For this review, take the finished solid that the model builds, in its own axes (mm). A direction names the side the tool comes from. Give positions to 0.01 mm unless a question says otherwise; leave off trailing zeros. Write each loop counter-clockwise with the first axis right and the second up, starting at its lowest first coordinate (ties: lowest second). Pieces come first, ordered by that corner, then holes.
Q1. Machinability: for faces 5 (the flat face through (10, -12, 1)), 6 (the flat face through (5, -24, 1)), which of the approach directions +Z, -Z, +X, -X, +Y, -Y give a long, thin tool a straight path to every point of the face, cutting with its end or side? Answer none if there is none.
Q2. We need section B-B (z = 0.95). Write out the cut boundary in (x, y), then the cut area to 3 significant figures.
Q3. Mouldability with a two-part tool opening along Y and no side actions: class faces 1 (the flat face through (36, 14, 1)), 2 (the flat face through (48, 19, 1)), 3 (the cylindrical face through (5.914, -17.567, 1.479)), 4 (the flat face through (24, 24, 1)) as released by +Y, released by -Y, zero draft, split by the parting line, or undercut.
Q4. Insertion check: P1, Ø2.5, axis at x = 5, y = 19, coming from the +Z side; P2, Ø1.5, axis at y = -6.5, z = 1.5, coming from the +X side. Each pin has a flat end and moves straight along its axis. Give the tip position at first contact, or say it passes through.
Q5. We need section D-D (x = 5). Write out the cut boundary in (y, z).
Q6. We need section A-A (x = 43). Write out the cut boundary in (y, z).
Q7. We need section C-C (y = -19). Write out the cut boundary in (x, z).
Q8. For line 1 (Y direction, x = 5, z = 0.7); line 2 (Y direction, x = 43, z = 1.95); line 3 (X direction, y = 18, z = 2.5), list the stretches that pass through material, from the lowest coordinate up.
```python
from build123d import *

# Parameters (mm, degrees)
SKETCH_1_R      = 1.7
EXTRUDE_1_DEPTH = 3


with BuildPart() as part:
    # 草图1 → 凸台-拉伸1 (new body)
    with BuildSketch(Plane.XY):
        with BuildLine():
            Line((0, 0), (0, 24))
            Line((0, 24), (24, 24))
            Line((24, 24), (38, 24))
            Line((38, 24), (48, 24))
            Line((48, 24), (48, 14))
            Line((48, 14), (34, 14))
            Line((34, 14), (24, 14))
            ThreePointArc((24, 14), (14.100505063, 9.899494937), (10, 0))
            Line((10, 0), (10, -12))
            Line((10, -12), (10, -24))
            Line((10, -24), (0, -24))
            Line((0, -24), (0, -14))
            Line((0, -14), (0, 0))
        make_face()
        with Locations((43, 19)):
            Circle(SKETCH_1_R, mode=Mode.SUBTRACT)
        with Locations((5, -19)):
            Circle(SKETCH_1_R, mode=Mode.SUBTRACT)
        with Locations((5, 19)):
            Circle(SKETCH_1_R, mode=Mode.SUBTRACT)
    extrude(amount=EXTRUDE_1_DEPTH)


solid = part.part
```
Computed:
1. face 5: +Z, -Z, +X, -Y
1. face 6: +Z, -Z, +X, -X, -Y
2. outline: (0, -24) - (10, -24) - (10, 0) arc R14 cw to (24, 14) - (48, 14) - (48, 24) - (0, 24) - close; hole circle Ø3.4 at (5, -19); hole circle Ø3.4 at (5, 19); hole circle Ø3.4 at (43, 19)
2. area: 875 mm2
3. face 1: released by -Y
3. face 2: zero draft
3. face 3: undercut
3. face 4: released by +Y
4. P1: passes through
4. P2: stops at x = 10
5. outline: (-24, 0) - (-20.7, 0) - (-20.7, 3) - (-24, 3) - close; (-17.3, 0) - (17.3, 0) - (17.3, 3) - (-17.3, 3) - close; (20.7, 0) - (24, 0) - (24, 3) - (20.7, 3) - close
6. outline: (14, 0) - (17.3, 0) - (17.3, 3) - (14, 3) - close; (20.7, 0) - (24, 0) - (24, 3) - (20.7, 3) - close
7. outline: (0, 0) - (3.3, 0) - (3.3, 3) - (0, 3) - close; (6.7, 0) - (10, 0) - (10, 3) - (6.7, 3) - close
8. line 1: y = -24 to -20.7, -17.3 to 17.3, 20.7 to 24
8. line 2: y = 14 to 17.3, 20.7 to 24
8. line 3: x = 0 to 3.63, 6.37 to 41.63, 44.37 to 48
